from build123d import *

# Parameters (mm, degrees)
BOSS_EXTRUDE1_DEPTH             = 3
CUT_EXTRUDE1_DEPTH              = 17.286497475
CUT_EXTRUDE1_DEPTH_BACK         = 17.286497475
SUPPORT_HOLE_R                  = 2.5
EXTRUDE_THIN1_REACH             = 57.365
EXTRUDE_THIN1_DIRECTION_2_REACH = 57.365
CUT_EXTRUDE2_DEPTH              = 36.780581326
CUT_EXTRUDE2_DEPTH_BACK         = 36.780581326
SKETCH6_R                       = 2.5
CUT_EXTRUDE3_DEPTH              = 1.55


with BuildPart() as part:
    # Sketch3 → Boss-Extrude1 (new, symmetric)
    with BuildSketch(Plane(origin=(0, -50, 0), x_dir=(1, 0, 0), z_dir=(0, 1, 0))):
        Polygon((-4.5, 10), (-4.5, -10), (4.5, -10), (4.5, -6), (12.5, -3.5), (12.5, 3.5), (4.5, 6), (4.5, 10), align=None)
    extrude(amount=BOSS_EXTRUDE1_DEPTH, both=True)

    # Support_hole → Cut-Extrude1 (cut, two sides: drawn at the far end of the back side and taken through both)
    with BuildSketch(Plane(origin=(0, -50, 0), x_dir=(1, 0, 0), z_dir=(0, 1, 0)).offset(-CUT_EXTRUDE1_DEPTH_BACK)):
        with Locations(Location((9.5, 0, 0), (0, 0, 270))):
            Circle(SUPPORT_HOLE_R)
    extrude(amount=CUT_EXTRUDE1_DEPTH + CUT_EXTRUDE1_DEPTH_BACK, mode=Mode.SUBTRACT)

    # Extrude-Thin1: up to this face of the body (flat: up to its plane)
    extrude_thin1_end = Plane(part.part.faces().sort_by_distance((4.5, -50, 8))[0])
    # Sketch8 → Extrude-Thin1 (add, up to the picked face)
    with BuildSketch(Plane(origin=(0, 0, 0), x_dir=(0, 0, -1), z_dir=(1, 0, 0)), mode=Mode.PRIVATE) as extrude_thin1_sk1:
        Polygon((-10, -53), (-10, -82), (10, -82), (10, -53), (7.5, -53), (7.5, -79.5), (-7.5, -79.5), (-7.5, -53), align=None)
    extrude_thin1_tool1 = split(extrude(extrude_thin1_sk1.sketch, amount=EXTRUDE_THIN1_REACH, mode=Mode.PRIVATE), bisect_by=extrude_thin1_end, keep=Keep.BOTH, mode=Mode.PRIVATE)
    add(extrude_thin1_tool1.solids().sort_by(Axis((0, -67.5, 9.647722), (1, 0, 0)))[0])

    # Extrude-Thin1 direction 2: up to this face of the body (flat: up to its plane)
    extrude_thin1_direction_2_end = Plane(part.part.faces().sort_by_distance((-4.5, -50, 0))[0])
    # Sketch8 → Extrude-Thin1 direction 2 (add, up to the picked face)
    with BuildSketch(Plane(origin=(0, 0, 0), x_dir=(0, 0, -1), z_dir=(1, 0, 0)), mode=Mode.PRIVATE) as extrude_thin1_direction_2_sk1:
        Polygon((-10, -53), (-10, -82), (10, -82), (10, -53), (7.5, -53), (7.5, -79.5), (-7.5, -79.5), (-7.5, -53), align=None)
    extrude_thin1_direction_2_tool1 = split(extrude(extrude_thin1_direction_2_sk1.sketch, amount=-EXTRUDE_THIN1_DIRECTION_2_REACH, mode=Mode.PRIVATE), bisect_by=extrude_thin1_direction_2_end, keep=Keep.BOTH, mode=Mode.PRIVATE)
    add(extrude_thin1_direction_2_tool1.solids().sort_by(Axis((0, -67.5, 9.647722), (-1, 0, 0)))[0])

    # Sketch6 → Cut-Extrude2 (cut, two sides: drawn at the far end of the back side and taken through both)
    with BuildSketch(Plane(origin=(0, -50, 0), x_dir=(1, 0, 0), z_dir=(0, 1, 0)).offset(-CUT_EXTRUDE2_DEPTH_BACK)):
        with Locations(Location((0, 0, 0), (0, 0, 270))):
            Circle(SKETCH6_R)
    extrude(amount=CUT_EXTRUDE2_DEPTH + CUT_EXTRUDE2_DEPTH_BACK, mode=Mode.SUBTRACT)

    # Sketch7 → Cut-Extrude3 (cut, symmetric)
    with BuildSketch(Plane(origin=(0, -50, 0), x_dir=(1, 0, 0), z_dir=(0, 1, 0))):
        Polygon((2.020725942, -3.5), (4.041451884, 0), (2.020725942, 3.5), (-2.020725942, 3.5), (-4.041451884, 0), (-2.020725942, -3.5), align=None)
    extrude(amount=CUT_EXTRUDE3_DEPTH, both=True, mode=Mode.SUBTRACT)


solid = part.part
Can you work these out from the model? Positions are in its coordinate system, mm. A direction names the side the tool comes from. Round coordinates to 2 decimals unless told otherwise and drop trailing zeros. Write each loop counter-clockwise with the first axis right and the second up, starting at its lowest first coordinate (ties: lowest second). Pieces come first, ordered by that corner, then holes. Notation, with made-up numbers: (-12.75, 48) - (38.25, 48) arc R33 ccw to (38.25, 84) - close; hole circle Ø2 at (53.5, 65). An arc over 180 degrees is marked (long way). Write each question's results on one line, items separated by ' | '. Start each with the question number.
1) Suppose I cut it at D-D (y = -67.5). List the corners of the cut face in (x, z) for me.
2) Suppose I cut it at A-A (z = 4.5). List the corners of the cut face in (x, y) for me.
3) Please list where these lines run through material, in increasing order: line 1 (X direction, y = -52.6, z = 0); line 2 (Y direction, x = -2.5, z = 1.5); line 3 (Z direction, x = 4, y = -69).
4) For pin 1 Ø10 at (y, z) = (-72.5, 4) entering from +X, with a flat end and sliding along its axis, tell me the tip position at first contact or that it passes through.
5) Suppose I cut it at B-B (y = -49.5). List the corners of the cut face in (x, z) for me.
6) We'd pull the mould along Y, two halves only. Please class faces 4 (the flat face through (3, -51.55, 0)), 5 (the cylindrical face through (7.06, -50.04, -0.54)), 6 (the flat face through (-2, -82, 2)): released by +Y, released by -Y, zero draft, split by the parting line, or undercut.
7) Which directions (+Z, -Z, +X, -X, +Y, -Y) give clear straight access to the entire face, cutting with the end or side of a thin tool? Please do faces 1 (the cylindrical face through (-2.44, -52.29, -0.54)), 2 (the flat face through (-3, -50, -1.8)), 3 (the flat face through (2, -79.5, -2)).
8) Suppose I cut it at C-C (x = 0). List the corners of the cut face in (y, z) for me, and give its area (3 significant figures).
Here are the results:
1) outline: (-4.5, -10) - (4.5, -10) - (4.5, -7.5) - (-4.5, -7.5) - close; (-4.5, 7.5) - (4.5, 7.5) - (4.5, 10) - (-4.5, 10) - close
2) outline: (-4.5, -82) - (4.5, -82) - (4.5, -79.5) - (-4.5, -79.5) - close; (-4.5, -53) - (9.3, -53) - (9.3, -47) - (-4.5, -47) - close
3) line 1: x = -4.5 to -2.5, 2.5 to 7, 12 to 12.5 | line 2: y = -82 to -79.5, -53 to -51.55, -48.45 to -47 | line 3: z = -10 to -7.5, 7.5 to 10
4) pin 1: stops at x = 4.5
5) outline: (-4.5, -10) - (4.5, -10) - (4.5, -6) - (12.5, -3.5) - (12.5, 3.5) - (4.5, 6) - (4.5, 10) - (-4.5, 10) - close; hole (-4.04, 0) - (-2.02, -3.5) - (2.02, -3.5) - (4.04, 0) - (2.02, 3.5) - (-2.02, 3.5) - close; hole circle Ø5 at (9.5, 0)
6) face 4: undercut | face 5: zero draft | face 6: released by -Y
7) face 1: +Y, -Y | face 2: none | face 3: +X, -X
8) outline: (-82, -10) - (-47, -10) - (-47, -2.5) - (-48.45, -2.5) - (-48.45, -3.5) - (-51.55, -3.5) - (-51.55, -2.5) - (-53, -2.5) - (-53, -7.5) - (-79.5, -7.5) - (-79.5, -2.5) - (-82, -2.5) - close; (-82, 2.5) - (-79.5, 2.5) - (-79.5, 7.5) - (-53, 7.5) - (-53, 2.5) - (-51.55, 2.5) - (-51.55, 3.5) - (-48.45, 3.5) - (-48.45, 2.5) - (-47, 2.5) - (-47, 10) - (-82, 10) - close | area: 254 mm2
